CAD build for the part. Positions are in the model's coordinates, mm. A direction names the side the tool comes from. Coordinates: 2 decimals unless noted, no trailing zeros. Loops run counter-clockwise (first coordinate to the right, second up) from the corner with the lowest first, then second, coordinate; pieces in that order, holes last. Notation, with made-up numbers: (67.5, -32) -> (115.5, -32) arc R21 ccw to (115.5, 0) -> close; hole circle Ø3 at (37, 21.25). An arc over 180 degrees is marked (long way). Write item = value, one per line. Start each with the question number.
(1) Band-saw the part on B-B (z = -13). Write the cut outline in (x, y), and give its area (3 significant figures).
(2) Band-saw the part on A-A (y = 3.5). Write the cut outline in (x, z), and give its area (3 significant figures).
(3) Band-saw the part on C-C (x = 39). Write the cut outline in (y, z), and give its area (3 significant figures).
(4) Tool access for faces 5 (the face through (1, 4, -9)), 6 (the face through (64.4, 6.27, -1.57)), 7 (the face through (33, 6, -32)): list every direction of +Z, -Z, +X, -X, +Y, -Y with a clear straight run to the whole face (end or side of a thin tool).
(5) Drill centre lines: line 1 (Z direction, x = 39.5, y = 6.75); line 2 (X direction, y = 4.25, z = -3.5); line 3 (Z direction, x = 42, y = 3.75). Where is each one in solid material? Low to high. Write a range as from..to.
(6) Flat gauge pins, fed straight in: P1, Ø3, axis at y = 5.5, z = -6.5, coming from the -X side; P2, Ø2, axis at x = 20, z = -9, coming from the +Y side; P3, Ø2, axis at y = 4.5, z = -12.5, coming from the +X side; P4, Ø3, axis at y = 4, z = -21.5, coming from the -X side. Where does each tip first touch, or does it go through?
(7) Pull direction X, two halves, no side cores. Call faces 1 (the face through (32.8, 5, -32.4)), 2 (the face through (33, 4, -31)), 3 (the face through (1, 6, -27)), 4 (the face through (2, 1, -16)): +X half, -X half, draft (parallel to the pull), parting line (faces both ways), or undercut.
(8) Band-saw the part on D-D (y = 6.5). Write the cut outline in (x, z), and give its area (3 significant figures).
```python
from build123d import *

# Parameters (mm, degrees)
SKETCH1_W           = 66
SKETCH1_H           = 33
BOSS_EXTRUDE1_DEPTH = 5
SKETCH2_W           = 64
SKETCH2_H           = 31
BOSS_EXTRUDE2_DEPTH = 2.5
SKETCH3_W           = 62
SKETCH3_H           = 29
CUT_EXTRUDE1_DEPTH  = 7
FILLET1_R           = 2
FILLET2_R           = 2
SKETCH4_W           = 12
SKETCH4_H           = 2.5
CUT_EXTRUDE2_DEPTH  = 7
SKETCH10_W          = 12
SKETCH10_H          = 3
CUT_EXTRUDE3_DEPTH  = 7
SKETCH11_W          = 15
SKETCH11_H          = 2.5
CUT_EXTRUDE4_DEPTH  = 7
SKETCH12_W          = 15
SKETCH12_H          = 3.5
CUT_EXTRUDE5_DEPTH  = 7


with BuildPart() as part:
    # Sketch1 → Boss-Extrude1 (new body)
    with BuildSketch(Plane(origin=(0, 0, 0), x_dir=(1, 0, 0), z_dir=(0, 1, 0))):
        with Locations((33, 16.5)):
            Rectangle(SKETCH1_W, SKETCH1_H)
    extrude(amount=BOSS_EXTRUDE1_DEPTH)

    # Sketch2 → Boss-Extrude2 (add)
    with BuildSketch(Plane(origin=(0, 5, 0), x_dir=(1, 0, 0), z_dir=(0, 1, 0))):
        with Locations((33, 16.5)):
            Rectangle(SKETCH2_W, SKETCH2_H)
    extrude(amount=BOSS_EXTRUDE2_DEPTH)

    # Sketch3 → Cut-Extrude1 (cut)
    with BuildSketch(Plane(origin=(0, 7.5, 0), x_dir=(1, 0, 0), z_dir=(0, 1, 0))):
        with Locations((33, 16.5)):
            Rectangle(SKETCH3_W, SKETCH3_H)
    extrude(amount=-CUT_EXTRUDE1_DEPTH, mode=Mode.SUBTRACT)

    # Fillet1
    fillet1_edges = [part.edges().sort_by_distance(p)[0] for p in [
        (33, 0, -33),
        (66, 0, -16.5),
        (33, 0, 0),
        (0, 0, -16.5),
        (0, 2.5, -33),
        (66, 2.5, -33),
        (66, 2.5, 0),
        (0, 2.5, 0),
    ]]
    fillet(fillet1_edges, radius=FILLET1_R)

    # Fillet2
    fillet2_edges = [part.edges().sort_by_distance(p)[0] for p in [
        (1, 6.25, -32),
        (1, 6.25, -1),
        (65, 6.25, -1),
        (65, 6.25, -32),
    ]]
    fillet(fillet2_edges, radius=FILLET2_R)

    # Sketch4 → Cut-Extrude2 (cut)
    with BuildSketch(Plane(origin=(65, 0, 0), x_dir=(0, 0, -1), z_dir=(1, 0, 0))):
        with Locations((16.5, 6.25)):
            Rectangle(SKETCH4_W, SKETCH4_H)
    extrude(amount=-CUT_EXTRUDE2_DEPTH, mode=Mode.SUBTRACT)

    # Sketch10 → Cut-Extrude3 (cut)
    with BuildSketch(Plane(origin=(66, 0, 0), x_dir=(0, 0, -1), z_dir=(1, 0, 0))):
        with Locations((16.5, 3.5)):
            Rectangle(SKETCH10_W, SKETCH10_H)
    extrude(amount=-CUT_EXTRUDE3_DEPTH, mode=Mode.SUBTRACT)

    # Sketch11 → Cut-Extrude4 (cut)
    with BuildSketch(Plane.ZY.offset(-1)):
        with Locations((-16.5, 6.25)):
            Rectangle(SKETCH11_W, SKETCH11_H)
    extrude(amount=-CUT_EXTRUDE4_DEPTH, mode=Mode.SUBTRACT)

    # Sketch12 → Cut-Extrude5 (cut)
    with BuildSketch(Plane.ZY):
        with Locations((-16.5, 3.25)):
            Rectangle(SKETCH12_W, SKETCH12_H)
    extrude(amount=-CUT_EXTRUDE5_DEPTH, mode=Mode.SUBTRACT)


solid = part.part
```
Findings below:
q1.outline = (0.06, 1.5) arc R2 ccw to (2, 0) -> (64, 0) arc R2 ccw to (66, 2) -> (64, 2) -> (64, 0.5) -> (2, 0.5) -> (2, 1.5) -> close
q1.area = 36.3 mm²
q2.outline = (0, -31) arc R2 ccw to (2, -33) -> (64, -33) arc R2 ccw to (66, -31) -> (66, -22.5) -> (64, -22.5) -> (64, -31) -> (2, -31) -> (2, -24) -> (0, -24) -> close; (0, -9) -> (2, -9) -> (2, -2) -> (64, -2) -> (64, -10.5) -> (66, -10.5) -> (66, -2) arc R2 ccw to (64, 0) -> (2, 0) arc R2 ccw to (0, -2) -> close
q2.area = 323 mm²
q3.outline = (0, -31) arc R2 ccw to (2, -33) -> (5, -33) -> (5, -32) -> (7.5, -32) -> (7.5, -31) -> (0.5, -31) -> (0.5, -2) -> (7.5, -2) -> (7.5, -1) -> (5, -1) -> (5, 0) -> (2, 0) arc R2 ccw to (0, -2) -> close
q3.area = 37.8 mm²
q4.face_5 = -X, +Y
q4.face_6 = +Z, +X, +Y
q4.face_7 = -Z, +X, -X, +Y
q5.line_1 = -32..-31, -2..-1
q5.line_2 = 0..2, 64..66
q5.line_3 = -33..-31, -2..0
q6.P1 = 0
q6.P2 = 0.5
q6.P3 = through
q6.P4 = 64
q7.face_1 = draft
q7.face_2 = undercut
q7.face_3 = -X half
q7.face_4 = undercut
q8.outline = (1, -30) arc R2 ccw to (3, -32) -> (63, -32) arc R2 ccw to (65, -30) -> (65, -22.5) -> (64, -22.5) -> (64, -31) -> (2, -31) -> (2, -24) -> (1, -24) -> close; (1, -9) -> (2, -9) -> (2, -2) -> (64, -2) -> (64, -10.5) -> (65, -10.5) -> (65, -3) arc R2 ccw to (63, -1) -> (3, -1) arc R2 ccw to (1, -3) -> close
q8.area = 156 mm²
